Autodesk Inventor part; units mm, degrees
ref_plane "YZ Plane" through (0, 0, 0) normal (1, 0, 0) x (0, 1, 0)
ref_plane "XZ Plane" through (0, 0, 0) normal (0, 1, 0) x (-1, 0, 0)
ref_plane "XY Plane" through (0, 0, 0) normal (0, 0, 1) x (1, 0, 0)
sketch "스케치1" plane through (0, 0, 0) normal (0, 1, 0) x (-1, 0, 0)
  circle A0 centre (12, 0) radius 5.5
  circle A1 centre (-12, 0) radius 5.5
  line L0 (30.1, 0) -> (-30.1, 0)
  line L1 (12, 0) -> (-12, 0) construction
  line L2 (12, 9.5) -> (-12, 9.5)
  line L3 (-12, -9.5) -> (12, -9.5)
  arc A2 (12, -9.5) -> (12, 9.5) centre (12, 0) ccw
  arc A3 (-12, 9.5) -> (-12, -9.5) centre (-12, 0) ccw
  point P0 (0, 0)
  point P1 (0, 0)
  dimension "d0" = 11
  dimension "d1" = 11
  dimension "d2" = 12
  dimension "d3" = 12
  dimension "d4" = 4
extrude "돌출1" add sketch "스케치1" along normal blind 15 contours L0 A2 L3 A3 A1 A0 | A0 L0 A1 A3 L2 A2
sketch "스케치2" plane through (0, 15, 0) normal (0, 1, 0) x (1, 0, 0)
  line L0 (-12, -9.5) -> (12, -9.5)
  line L1 (0, -9.5) -> (-23, -9.5)
  line L2 (0, -9.5) -> (23, -9.5)
  line L3 (-21.5, 10.5) -> (21.5, 10.5)
  line L4 (-36.4, 0) -> (36.4, 0)
  line L5 (0, 14.5) -> (0, -13.5)
  line L6 (0, -9.5) -> (0, 10.5)
  line L7 (-21.5, 10.5) -> (-23, -9.5)
  line L8 (21.5, 10.5) -> (23, -9.5)
  line L9 (-23, -9.5) -> (-26, -9.5)
  line L10 (23, -9.5) -> (26, -9.5)
  line L11 (-21.5, 10.5) -> (-24.5, 10.5)
  line L12 (-24.5, 10.5) -> (-26, -9.5)
  line L13 (21.5, 10.5) -> (24.5, 10.5)
  line L14 (24.5, 10.5) -> (26, -9.5)
  point P0 (0, 0)
  dimension "d7" = 23
  dimension "d8" = 23
  dimension "d9" = 43
  dimension "d10" = 20
  dimension "d11" = 3
  dimension "d12" = 3
  dimension "d13" = 3
  dimension "d14" = 3
extrude "돌출2" add sketch "스케치2" along normal blind 3
sketch "스케치3" plane through (0, 18, 0) normal (0, 1, 0) x (1, 0, 0)
  line L0 (-21.5, 10.5) -> (-23, -9.5)
  line L1 (21.5, 10.5) -> (23, -9.5)
  line L2 (-26, -9.5) -> (26, -9.5)
  line L3 (26, -9.5) -> (24.5, 10.5)
  line L4 (24.5, 10.5) -> (-24.5, 10.5)
  line L5 (-24.5, 10.5) -> (-26, -9.5)
  point P0 (0, 0)
  point P1 (23, -9.5)
  point P2 (-23, -9.5)
extrude "돌출3" add sketch "스케치3" along normal blind 18 contours L0 L2 L5 L4 | L4 L3 L2 L1
sketch "스케치4" plane through (0, 36, 0) normal (0, 1, 0) x (1, 0, 0)
  line L0 (23, -9.5) -> (21.5, 10.5)
  line L1 (21.5, 10.5) -> (-21.5, 10.5)
  line L2 (-21.5, 10.5) -> (-23, -9.5)
  line L3 (-23, -9.5) -> (23, -9.5)
  line L4 (-22.2875, 0) -> (22.2875, 0)
  line L5 (-26, -9.5) -> (-23, -9.5)
  line L6 (-23, -9.5) -> (-21.5, 10.5)
  line L7 (-21.5, 10.5) -> (-24.5, 10.5)
  line L8 (-24.5, 10.5) -> (-26, -9.5)
  line L9 (24.5, 10.5) -> (21.5, 10.5)
  line L10 (21.5, 10.5) -> (23, -9.5)
  line L11 (23, -9.5) -> (26, -9.5)
  line L12 (26, -9.5) -> (24.5, 10.5)
  point P0 (0, 0)
  point P1 (0, 0)
extrude "돌출4" add sketch "스케치4" along normal blind 3 contours L0 L9 L12 L11 | L4 L2 L1 L0 | L5 L8 L7 L2
properties part number "카메라 상단"
Read the model definition and answer for the solid it produces. Units are mm, in the model's axes. A direction names the side the tool comes from. Round coordinates to 2 decimals unless told otherwise and drop trailing zeros. Write each loop counter-clockwise with the first axis right and the second up, starting at its lowest first coordinate (ties: lowest second). Pieces come first, ordered by that corner, then holes.
1. The part is cut by section C-C, the plane z = -4.75. Determine the outline of the cut face in (x, y).
2. The part is cut by section B-B, the plane y = 23.5. Determine the outline of the cut face in (x, z).
3. The part is cut by section A-A, the plane x = 3. Determine the outline of the cut face in (y, z), then the cut area to 4 significant figures.
4. The part is cut by section D-D, the plane z = 2.25. Determine the outline of the cut face in (x, y).
5. Straight lines are drawn through the part: L1, parallel to X at y = 10, z = 0; L2, parallel to Z at x = -12, y = 11; L3, parallel to Y at x = -1.5, z = -2.5. For each, find the intervals that lie inside material, in ascending order.
6. Given pin 1 Ø1.5 at (y, z) = (8, 2.5) entering from +X; pin 2 Ø8 at (y, z) = (13, 2) entering from +X; pin 3 Ø0.9 at (x, y) = (-8, 38) entering from +Z, each flat-ended and moving along its own axis, determine where each tip first touches the part or whether it passes through.
7. Determine the mould class of faces 5 (the face through (0, 0, 0)), 6 (the face through (-21.498, 7.395, 0.209)), 7 (the face through (22.24, 28.35, -0.64)) for opening direction X: pulls with the +X half, pulls with the -X half, needs draft (parallel to the pull), parting line crosses it, or undercut.
8. Which of the six approach directions +Z, -Z, +X, -X, +Y, -Y give full straight-line access (tool end or side, diameter ignored) to faces 1 (the face through (6.92, 7.4, 2.11)), 2 (the face through (-22.24, 28.35, -0.64)), 3 (the face through (0, 7, -9.5)), 4 (the face through (0, 37, 0))?
Values:
1. outline: (-24.93, 15) - (-20.23, 15) - (-20.23, 0) - (-14.77, 0) - (-14.77, 15) - (-9.23, 15) - (-9.23, 0) - (9.23, 0) - (9.23, 15) - (14.77, 15) - (14.77, 0) - (20.23, 0) - (20.23, 15) - (24.93, 15) - (24.93, 39) - (-24.93, 39) - close; hole (-21.93, 18) - (21.93, 18) - (21.93, 36) - (-21.93, 36) - close
2. outline: (-26, 9.5) - (-24.5, -10.5) - (-21.5, -10.5) - (-23, 9.5) - close; (21.5, -10.5) - (24.5, -10.5) - (26, 9.5) - (23, 9.5) - close
3. outline: (0, -9.5) - (15, -9.5) - (15, -10.5) - (18, -10.5) - (18, 9.5) - (0, 9.5) - close; (36, -10.5) - (39, -10.5) - (39, 0) - (36, 0) - close
3. area: 376.5 mm2
4. outline: (-25.46, 15) - (-21.23, 15) - (-21.23, 0) - (-17.02, 0) - (-17.02, 15) - (-6.98, 15) - (-6.98, 0) - (6.98, 0) - (6.98, 15) - (17.02, 15) - (17.02, 0) - (21.23, 0) - (21.23, 15) - (25.46, 15) - (25.46, 39) - (22.46, 39) - (22.46, 18) - (-22.46, 18) - (-22.46, 39) - (-25.46, 39) - close
5. L1: x = -21.5 to -17.5, -6.5 to 6.5, 17.5 to 21.5
5. L2: z = -9.5 to -5.5, 5.5 to 9.5
5. L3: y = 0 to 18, 36 to 39
6. pin 1: stops at x = 21.34
6. pin 2: stops at x = 25.7
6. pin 3: stops at z = 0
7. face 5: needs draft
7. face 6: pulls with the -X half
7. face 7: undercut
8. face 1: -Y
8. face 2: +Z
8. face 3: -Z, +X, -X, -Y
8. face 4: +Z, +Y
